Study the drawing (mm; zero at the part's minimum x, y, z) and answer. A direction names the side the tool comes from. Give positions to 0.01 mm unless a question says otherwise; leave off trailing zeros. Write each loop counter-clockwise with the first axis right and the second up, starting at its lowest first coordinate (ties: lowest second). Pieces come first, ordered by that corner, then holes. Notation, with made-up numbers: (62, 78) -> (82, 78) arc R23 ccw to (82, 88) -> close; hole circle Ø2 at (21.25, 3.5). An arc over 180 degrees is marked (long way). Use CSV: the item, a comma, the result in double quotes. Start each with the question number.
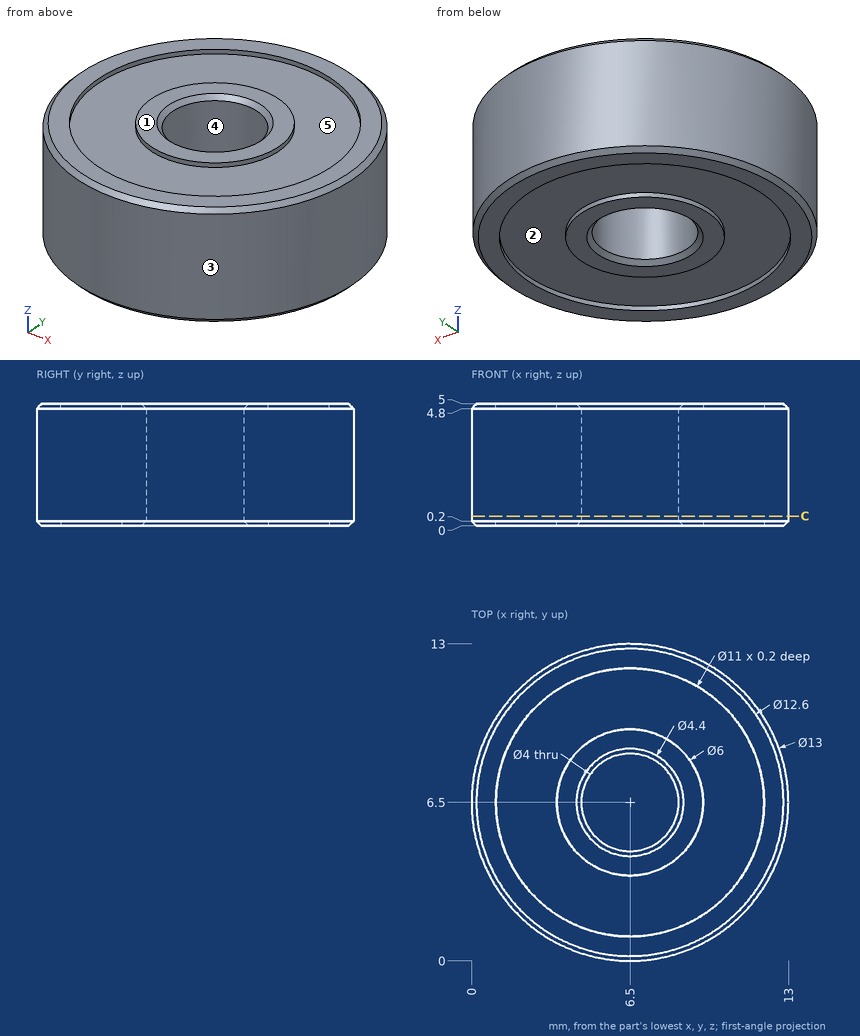
Q1. The mould has two halves that part along X. Classify the marked faces 1, 2 and 3: +X half, -X half, draft (parallel to the pull), parting line (faces both ways), or undercut.
Q2. Section C-C on z = 0.4 is taken. Give the vertices of the cut face in (x, y), then the cut area to 3 significant figures.
Q3. Straight lines are drawn through the part: L1, parallel to Y at x = 6.5, z = 3.85; L2, parallel to Y at x = 6.5, z = 4.9; L3, parallel to Y at x = 6.5, z = 0.15. For each, find the intervals that lie inside material, in ascending order.
Q4. Flat-ended cylindrical pins translate along their axes: pin 1 Ø1 at (y, z) = (10, 2.5) entering from -X; pin 2 Ø2.5 at (x, y) = (6.5, 6.5) entering from +Z; pin 3 Ø2 at (y, z) = (4, 1) entering from +X; pin 4 Ø1.5 at (x, z) = (10.5, 3) entering from -Y. Find the tip coordinate at first contact, or state that the pin passes through.
Q5. For the marked faces 4 and 5, determine the directions among +Z, -Z, +X, -X, +Y, -Y from which every point of the face is accessible in a straight line to the end or side of a thin tool.
Output:
1,face 1,"draft"
1,face 2,"undercut"
1,face 3,"parting line"
2,outline,"circle Ø13 at (6.5, 6.5); hole circle Ø4 at (6.5, 6.5)"
2,area,"120 mm²"
3,L1,"0 to 4.5, 8.5 to 13"
3,L2,"0.1 to 1, 3.5 to 4.4, 8.6 to 9.5, 12 to 12.9"
3,L3,"0.05 to 1, 3.5 to 4.45, 8.55 to 9.5, 12 to 12.95"
4,pin 1,"x = 0.73"
4,pin 2,"through"
4,pin 3,"x = 12.82"
4,pin 4,"y = 0.87"
5,face 4,"+Z, -Z"
5,face 5,"+Z"
